from build123d import *

# Parameters (mm, degrees)
CROQUIS1_R              = 0.9
CROQUIS1_R_2            = 1.1
SALIENTE_EXTRUIR1_DEPTH = 6.5
CORTAR_EXTRUIR6_DEPTH   = 4.5
CHAFL_N1_SIZE           = 1
CHAFL_N1_SIZE_2         = 0.742384029
CROQUIS5_W              = 12
CROQUIS5_H              = 2.5
CORTAR_EXTRUIR7_DEPTH   = 3
CROQUIS6_R              = 2.25
CORTAR_EXTRUIR8_DEPTH   = 2.9
CHAFL_N3_SIZE           = 0.2
CROQUIS7_R              = 4
CORTAR_EXTRUIR9_DEPTH   = 23.5
CHAFL_N2_SIZE           = 1
CORTAR_EXTRUIR2_START   = -6.5
CROQUIS3_W              = 6
CROQUIS3_H              = 17.049295702
CORTAR_EXTRUIR2_DEPTH   = 3
CROQUIS8_W              = 10.359823846
CROQUIS8_H              = 13.918607014
CORTAR_EXTRUIR10_DEPTH  = 5.5


with BuildPart() as part:
    # Croquis1 → Saliente-Extruir1 (new body)
    with BuildSketch(Plane.XY):
        with BuildLine():
            Line((-1.326649916, 8), (20, 8))
            Line((20, 8), (20, 0))
            Line((20, 0), (8, 0))
            Line((8, 0), (-8.109253973, 0))
            ThreePointArc((-8.109253973, 0), (-6.185391706, 5.24413286), (-1.326649916, 8))
        make_face()
        with Locations(Location((0, 6, 0), (0, 0, 180))):
            Circle(CROQUIS1_R, mode=Mode.SUBTRACT)
        with Locations(Location((12, 3.5, 0), (0, 0, 180))):
            Circle(CROQUIS1_R_2, mode=Mode.SUBTRACT)
    extrude(amount=SALIENTE_EXTRUIR1_DEPTH)

    # Croquis4 → Cortar-Extruir6 (cut)
    with BuildSketch(Plane(origin=(0, 0, 0), x_dir=(-1, 0, 0), z_dir=(0, 0, -1))):
        with BuildLine():
            Line((-5.656854249, 7), (-8, 4.123105626))
            Line((-8, 4.123105626), (-8, 0))
            Line((-8, 0), (8.109253973, 0))
            Line((8.109253973, 0), (9, 0))
            ThreePointArc((9, 0), (3.878679656, 8.121320344), (-5.656854249, 7))
        make_face()
    extrude(amount=-CORTAR_EXTRUIR6_DEPTH, mode=Mode.SUBTRACT)

    # Chaflán1
    # the kernel refuses this chamfer: 1, 0.742384029 mm, written as the material it takes off along each edge
    with BuildSketch(Plane(origin=(-5.698510996, 8, 6.5), x_dir=(0, 0, -1), z_dir=(1, 0, 0))) as chafl_n1_piece_1:
        Polygon((CHAFL_N1_SIZE, 0), (0, -CHAFL_N1_SIZE), (0, 0), align=None)
    extrude(amount=28.270193984, mode=Mode.SUBTRACT)
    with BuildSketch(Plane(origin=(4.123105626, 8, 4.5), x_dir=(1, 0, 0), z_dir=(0, 0, -1))) as chafl_n1_piece_2:
        with BuildLine():
            Line((CHAFL_N1_SIZE_2, 0), (0.916025454, 0.542979283))
            ThreePointArc((0.916025454, 0.542979283), (0.478949419, 0.265590562), (0, 0))
            Line((0, 0), (CHAFL_N1_SIZE_2, 0))
        make_face()
    extrude(amount=7.23772815, mode=Mode.SUBTRACT)
    with BuildSketch(Plane(origin=(0, 0, 6.5), x_dir=(-0.9501026430594787, -0.31193744188762096, 0), z_dir=(0.31193744188762096, -0.9501026430594787, 0))) as chafl_n1_piece_3:
        Polygon((8.109253973 - CHAFL_N1_SIZE, 0), (8.109253973, CHAFL_N1_SIZE), (8.109253973, 0), align=None)
    revolve(axis=Axis((0, 0, 6.5), (0, 0, -1)), revolution_arc=116.936314038, mode=Mode.SUBTRACT)

    # Croquis5 → Cortar-Extruir7 (cut)
    with BuildSketch(Plane(origin=(0, 0, 0), x_dir=(-1, 0, 0), z_dir=(0, 0, -1))):
        with Locations((-14, 1.25)):
            Rectangle(CROQUIS5_W, CROQUIS5_H)
    extrude(amount=-CORTAR_EXTRUIR7_DEPTH, mode=Mode.SUBTRACT)

    # Croquis6 → Cortar-Extruir8 (cut)
    with BuildSketch(Plane.XY.offset(6.5)):
        with Locations((12, 3.5)):
            Circle(CROQUIS6_R)
    extrude(amount=-CORTAR_EXTRUIR8_DEPTH, mode=Mode.SUBTRACT)

    # Chaflán3
    chafl_n3_edges = [part.edges().sort_by_distance(p)[0] for p in [
        (0.9, 6, 4.5),
    ]]
    chamfer(chafl_n3_edges, length=CHAFL_N3_SIZE)

    # Simetría1: part across plane


with BuildPart() as part_1:
    add(part.part)
    add(part.part.mirror(Plane(origin=(20, 0, 6.5), x_dir=(0, 0, 1), z_dir=(0, 1, 0))))

    # Croquis7 → Cortar-Extruir9 (cut, through all)
    with BuildSketch(Plane.XY.offset(6.5)):
        Circle(CROQUIS7_R)
    extrude(amount=-CORTAR_EXTRUIR9_DEPTH, mode=Mode.SUBTRACT)

    # Chaflán2
    chafl_n2_edges = [part_1.edges().sort_by_distance(p)[0] for p in [
        (-4, 0, 6.5),
    ]]
    chamfer(chafl_n2_edges, length=CHAFL_N2_SIZE)

    # Simetría2: part across plane


with BuildPart() as part_2:
    add(part_1.part)
    add(part_1.part.mirror(Plane(origin=(20, 8, 6.5), x_dir=(0, 0, 1), z_dir=(-1, 0, 0))))

    # Croquis3 → Cortar-Extruir2 (cut)
    with BuildSketch(Plane.XY.offset(6.5).offset(CORTAR_EXTRUIR2_START)):
        with Locations((20, -8)):
            Rectangle(CROQUIS3_W, CROQUIS3_H)
    extrude(amount=CORTAR_EXTRUIR2_DEPTH, mode=Mode.SUBTRACT)

    # Croquis8 → Cortar-Extruir10 (cut)
    with BuildSketch(Plane(origin=(0, 0, 0), x_dir=(-1, 0, 0), z_dir=(0, 0, -1))):
        with Locations((-20, 0)):
            Rectangle(CROQUIS8_W, CROQUIS8_H)
    extrude(amount=-CORTAR_EXTRUIR10_DEPTH, mode=Mode.SUBTRACT)


solid = part_2.part
Geometry: final body of the model. Coordinates: model frame, mm. A direction names the side the tool comes from. Coordinates: 2 decimals unless noted, no trailing zeros. Loops run counter-clockwise (first coordinate to the right, second up) from the corner with the lowest first, then second, coordinate; pieces in that order, holes last. Notation, with made-up numbers: M 41,2.5 L 58,2.5 A23 cw 58,33.5 Z; hole C 67.25,16 d5. An arc over 180 degrees is marked long. One line per item, written item: value. Start each with the question number.
1) Pin query (flat end, axial travel): P1, Ø2, axis at x = 11.5, y = 4, coming from the +Z side; P2, Ø8, axis at x = -1.5, y = 0, coming from the -Z side; P3, Ø1.5, axis at x = 10, y = -1, coming from the -Z side. Return the tip coordinate at first contact, or that it passes through.
2) Reachability of faces 1 (the flat face through (33.188, -5.582, 2.218)), 2 (the flat face through (28, 5, 3.6)), 3 (the flat face through (10, -2.5, 1)), 4 (the flat face through (6.812, -5.582, 2.218)) from +Z, -Z, +X, -X, +Y, -Y: full face, straight path, thin tool, end or side. Return the list, or none.
3) Draft query along Y for faces 5 (the cylindrical face through (27.762, 4.574, 1.775)), 6 (the flat face through (17, -7.5, 1.5)), 7 (the cylindrical face through (11.492, 4.476, 1.775)), 8 (the conical face through (-7.28, 0.14, 6.33)). Return one class per face: released by +Y, released by -Y, zero draft, split by the parting line, or undercut.
4) Cut plane A-A (x = 40). Return loops of the section in (y, z), then the cut area to 3 significant figures.
5) Cut plane B-B (z = 2). Count the separate pieces of the cut face and the enclosed holes in it, then the cut area to 3 significant figures.
6) Material intervals for L1, parallel to X at y = 3.5, z = 1.8; L2, parallel to Y at x = 28, z = 5.25; L3, parallel to Y at x = 0, z = 5.5, sorted ascending. Write a range as from..to.
Evaluation:
1. P1: z = 3.6
1. P2: z = 4.5
1. P3: z = 3
2. face 1: -Z, +X
2. face 2: +Z
2. face 3: -Z, +X, -X
2. face 4: -Z, -X
3. face 5: undercut
3. face 6: zero draft
3. face 7: undercut
3. face 8: split by the parting line
4. outline: M -8,4.5 L -7.1,4.5 L -6.9,4.7 L -6.9,6.5 L -7,6.5 L -8,5.5 Z; M -5.1,4.7 L -4.9,4.5 L -4,4.5 L -4,5.5 L -5,6.5 L -5.1,6.5 Z; M 4,4.5 L 4.9,4.5 L 5.1,4.7 L 5.1,6.5 L 5,6.5 L 4,5.5 Z; M 6.9,4.7 L 7.1,4.5 L 8,4.5 L 8,5.5 L 7,6.5 L 6.9,6.5 Z
4. area: 6.72 mm^2
5. separate pieces: 3
5. enclosed holes: 0
5. area: 175 mm^2
6. L1: 8..10.9, 13.1..14.82, 25.18..26.9, 29.1..32
6. L2: -8..-5.75, -1.25..1.25, 5.75..8
6. L3: -8..-6.9, -5.1..-4, 4..5.1, 6.9..8
